```python
from build123d import *

# Parameters (mm, degrees)
SKETCH1_R           = 11
SKETCH1_R_2         = 1
BOSS_EXTRUDE1_DEPTH = 6
SKETCH2_R           = 4
CUT_EXTRUDE1_DEPTH  = 5.5


with BuildPart() as part:
    # Sketch1 → Boss-Extrude1 (new body)
    with BuildSketch(Plane(origin=(0, 0, 0), x_dir=(1, 0, 0), z_dir=(0, 1, 0))):
        with Locations(Location((0, 0, 0), (0, 0, 270))):
            Circle(SKETCH1_R)
        with Locations(Location((0, 8, 0), (0, 0, 270))):
            Circle(SKETCH1_R_2, mode=Mode.SUBTRACT)
        with Locations(Location((5.656854249, 5.656854249, 0), (0, 0, 270))):
            Circle(SKETCH1_R_2, mode=Mode.SUBTRACT)
        with Locations(Location((8, 0, 0), (0, 0, 270))):
            Circle(SKETCH1_R_2, mode=Mode.SUBTRACT)
        with Locations(Location((5.656854249, -5.656854249, 0), (0, 0, 270))):
            Circle(SKETCH1_R_2, mode=Mode.SUBTRACT)
        with Locations(Location((0, -8, 0), (0, 0, 270))):
            Circle(SKETCH1_R_2, mode=Mode.SUBTRACT)
        with Locations(Location((-5.656854249, -5.656854249, 0), (0, 0, 270))):
            Circle(SKETCH1_R_2, mode=Mode.SUBTRACT)
        with Locations(Location((-8, 0, 0), (0, 0, 270))):
            Circle(SKETCH1_R_2, mode=Mode.SUBTRACT)
        with Locations(Location((-5.656854249, 5.656854249, 0), (0, 0, 270))):
            Circle(SKETCH1_R_2, mode=Mode.SUBTRACT)
    extrude(amount=BOSS_EXTRUDE1_DEPTH)

    # Sketch2 → Cut-Extrude1 (cut)
    with BuildSketch(Plane.XZ):
        with Locations(Location((0, 0, 0), (0, 0, 270))):
            Circle(SKETCH2_R)
    extrude(amount=-CUT_EXTRUDE1_DEPTH, mode=Mode.SUBTRACT)


solid = part.part
```
The listing builds one solid part. Answer for the finished solid, in the listing's coordinates (mm). A direction names the side the tool comes from. Coordinates: 2 decimals unless noted, no trailing zeros. Write each loop counter-clockwise with the first axis right and the second up, starting at its lowest first coordinate (ties: lowest second). Pieces come first, ordered by that corner, then holes. Notation, with made-up numbers: (-14.5, 51.25) - (16.5, 51.25) arc R16 ccw to (16.5, 74.25) - close; hole circle Ø10 at (73.5, 44). An arc over 180 degrees is marked (long way). Return JSON: item names as keys, results as strings. Group by question number.
1. Given pin 1 (9 mm diameter, centred on x = 1.5, z = 0, fed in from -Y), flat-ended and moving along its own axis, determine where the tip first touches the part or whether it passes through.
2. A cutting plane is placed at D-D, the plane z = -8. Determine the outline of the cut face in (x, y), plus the area to 3 significant figures.
3. A cutting plane is placed at B-B, the plane x = 5. Determine the outline of the cut face in (y, z), plus the area to 3 significant figures.
4. Which of the six approach directions +Z, -Z, +X, -X, +Y, -Y give full straight-line access (tool end or side, diameter ignored) to faces 1 (the cylindrical face through (-10.74, 2.96, -2.38)), 2 (the cylindrical face through (-3.905, 2.712, 0.867))?
5. A cutting plane is placed at A-A, the plane z = 5. Determine the outline of the cut face in (x, y), plus the area to 3 significant figures.
6. A cutting plane is placed at C-C, the plane x = 7.5. Determine the outline of the cut face in (y, z), plus the area to 3 significant figures.
7. Straight lines are drawn through the part: L1, parallel to X at y = 3.05, z = 0; L2, parallel to Z at x = 6.5, y = 4.9; L3, parallel to Z at x = -0.5, y = 3.4. For each, find the intervals that lie inside material, in ascending order.
Ans:
{
 "1": {"pin 1": "y = 0"},
 "2": {"outline": "(-7.55, 0) - (-1, 0) - (-1, 6) - (-7.55, 6) - close; (1, 0) - (7.55, 0) - (7.55, 6) - (1, 6) - close", "area": "78.6 mm²"},
 "3": {"outline": "(0, -9.8) - (6, -9.8) - (6, -6.41) - (0, -6.41) - close; (0, -4.9) - (6, -4.9) - (6, 4.9) - (0, 4.9) - close; (0, 6.41) - (6, 6.41) - (6, 9.8) - (0, 9.8) - close", "area": "99.5 mm²"},
 "4": {"face 1": "+Y, -Y", "face 2": "-Y"},
 "5": {"outline": "(-9.8, 0) - (-6.41, 0) - (-6.41, 6) - (-9.8, 6) - close; (-4.9, 0) - (4.9, 0) - (4.9, 6) - (-4.9, 6) - close; (6.41, 0) - (9.8, 0) - (9.8, 6) - (6.41, 6) - close", "area": "99.5 mm²"},
 "6": {"outline": "(0, -8.05) - (6, -8.05) - (6, -0.87) - (0, -0.87) - close; (0, 0.87) - (6, 0.87) - (6, 8.05) - (0, 8.05) - close", "area": "86.2 mm²"},
 "7": {"L1": "-11 to -9, -7 to -4, 4 to 7, 9 to 11", "L2": "-8.87 to -6.19, -5.12 to 5.12, 6.19 to 8.87", "L3": "-10.99 to -8.87, -7.13 to -3.97, 3.97 to 7.13, 8.87 to 10.99"}
}
